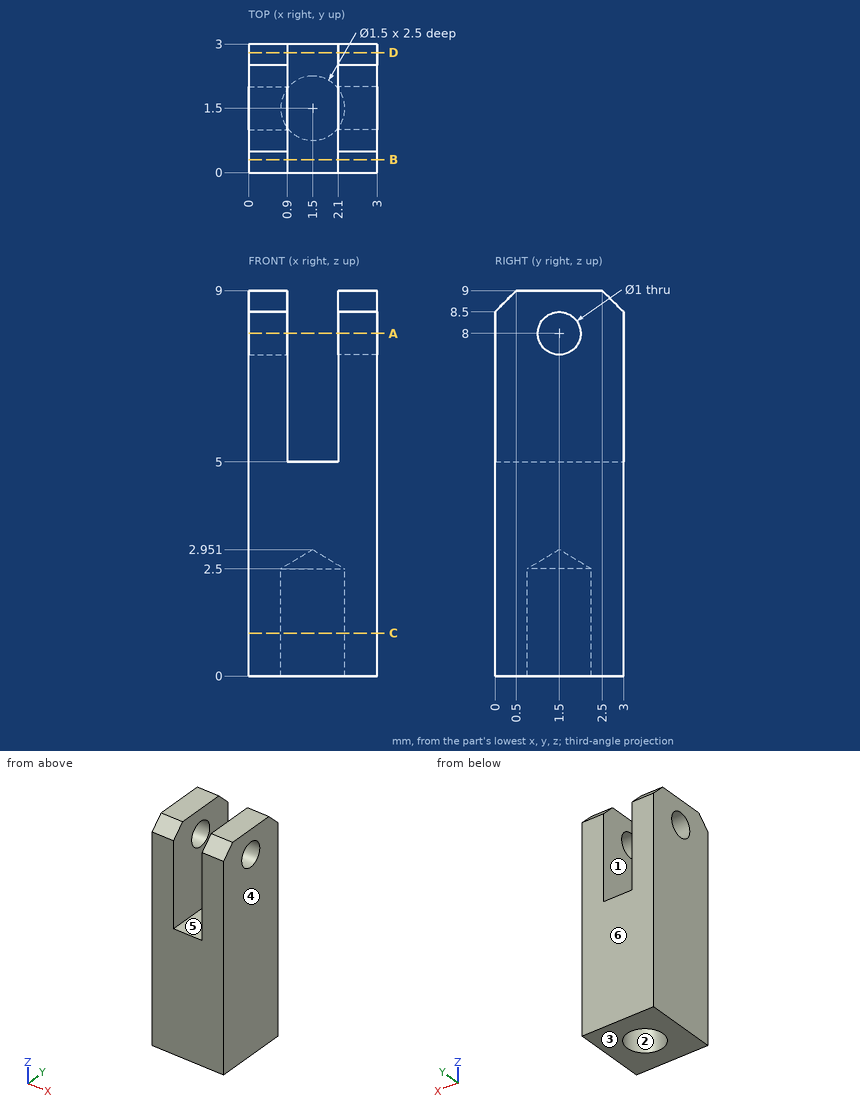
Could you check a few things on this drawing? It's one solid part, dimensions in mm from its lowest x, y, z. A direction names the side the tool comes from. Give positions to 0.01 mm unless a question says otherwise; leave off trailing zeros. Order: outer loops, then holes, each group sorted by start corner. A loop starts at its lowest first (then second) coordinate and runs counter-clockwise, first axis right, second up. Notation, with made-up numbers: M 80,-21.5 L 137,-21.5 A28 cw 137,17.5 Z; hole C 54,9 d10. An arc over 180 degrees is marked long. Use one line per item in the form item = value. Start each with the question number.
Item 1: If we section it at A-A (z = 8): Write out the boundary of the cut face in (x, y).
Item 2: For the marked faces 1, 2 and 3, which set-ups out of +Z, -Z, +X, -X, +Y, -Y let a thin tool reach every point of the face, with its end or its side?
Item 3: If we section it at B-B (y = 0.3): Write out the boundary of the cut face in (x, z).
Item 4: If I drill on line 1 along Y through (x, z) = (0.4, 8); line 2 along X through (y, z) = (1.8, 6.75); line 3 along X through (y, z) = (1.5, 1.1), over which ranges is the centre line in solid material (lowest first)?
Item 5: If we section it at D-D (y = 2.8): Write out the boundary of the cut face in (x, z).
Item 6: If we section it at C-C (z = 1): Write out the boundary of the cut face in (x, y).
Item 7: We'd pull the mould along X, two halves only. Please class the marked faces 4, 5 and 6: +X half, -X half, draft (parallel to the pull), parting line (faces both ways), or undercut.
Outcome:
q1.outline = M 0,0 L 0.9,0 L 0.9,1 L 0,1 Z; M 0,2 L 0.9,2 L 0.9,3 L 0,3 Z; M 2.1,0 L 3,0 L 3,1 L 2.1,1 Z; M 2.1,2 L 3,2 L 3,3 L 2.1,3 Z
q2.face_1 = +Z, +Y, -Y
q2.face_2 = -Z
q2.face_3 = -Z, +X, -X, +Y, -Y
q3.outline = M 0,0 L 3,0 L 3,8.8 L 2.1,8.8 L 2.1,5 L 0.9,5 L 0.9,8.8 L 0,8.8 Z
q4.line_1 = 0 to 1, 2 to 3
q4.line_2 = 0 to 0.9, 2.1 to 3
q4.line_3 = 0 to 0.75, 2.25 to 3
q5.outline = M 0,0 L 3,0 L 3,8.7 L 2.1,8.7 L 2.1,5 L 0.9,5 L 0.9,8.7 L 0,8.7 Z
q6.outline = M 0,0 L 3,0 L 3,3 L 0,3 Z; hole C 1.5,1.5 d1.5
q7.face_4 = +X half
q7.face_5 = undercut
q7.face_6 = draft
